```python
from build123d import *

# Parameters (mm, degrees)
F1_DEPTH = 3
F2_DEPTH = 6
F3_W     = 3
F3_H     = 2.9
F4_DEPTH = 1.5
F5_DEPTH = 3
F6_R     = 0.5


with BuildPart() as f1:
    # F0 (on Top) → F1 (new body)
    with BuildSketch(Plane.XY):
        with BuildLine():
            Line((-8.1, -17.1), (8.1, -17.1))
            ThreePointArc((8.1, -17.1), (14.463961, -14.463961), (17.1, -8.1))
            Line((17.1, -8.1), (17.1, 8.1))
            ThreePointArc((17.1, 8.1), (14.463961, 14.463961), (8.1, 17.1))
            Line((8.1, 17.1), (-8.1, 17.1))
            ThreePointArc((-8.1, 17.1), (-14.463961, 14.463961), (-17.1, 8.1))
            Line((-17.1, 8.1), (-17.1, -8.1))
            ThreePointArc((-17.1, -8.1), (-14.463961, -14.463961), (-8.1, -17.1))
        make_face()
        with BuildLine():
            ThreePointArc((14, -6.1), (12.974874, -8.574874), (10.5, -9.6))
            Line((10.5, -9.6), (-10.5, -9.6))
            ThreePointArc((-10.5, -9.6), (-12.974874, -8.574874), (-14, -6.1))
            Line((-14, -6.1), (-14, 0))
            Line((-14, 0), (-14, 8.1))
            ThreePointArc((-14, 8.1), (-12.242641, 12.342641), (-8, 14.1))
            Line((-8, 14.1), (8, 14.1))
            ThreePointArc((8, 14.1), (12.242641, 12.342641), (14, 8.1))
            Line((14, 8.1), (14, 0))
            Line((14, 0), (14, -6.1))
        make_face(mode=Mode.SUBTRACT)
    extrude(amount=F1_DEPTH)

    # F0 (on Top) → F2 (join)
    with BuildSketch(Plane.XY):
        with BuildLine():
            Line((-20, -20), (20, -20))
            Line((20, -20), (20, 9.5))
            ThreePointArc((20, 9.5), (16.924621, 16.924621), (9.5, 20))
            Line((9.5, 20), (-9.5, 20))
            ThreePointArc((-9.5, 20), (-16.924621, 16.924621), (-20, 9.5))
            Line((-20, 9.5), (-20, -20))
        make_face()
        with BuildLine():
            ThreePointArc((17.1, -8.1), (14.463961, -14.463961), (8.1, -17.1))
            Line((8.1, -17.1), (-8.1, -17.1))
            ThreePointArc((-8.1, -17.1), (-14.463961, -14.463961), (-17.1, -8.1))
            Line((-17.1, -8.1), (-17.1, 8.1))
            ThreePointArc((-17.1, 8.1), (-14.463961, 14.463961), (-8.1, 17.1))
            Line((-8.1, 17.1), (8.1, 17.1))
            ThreePointArc((8.1, 17.1), (14.463961, 14.463961), (17.1, 8.1))
            Line((17.1, 8.1), (17.1, -8.1))
        make_face(mode=Mode.SUBTRACT)
    extrude(amount=F2_DEPTH)

    # F3 (on face) → F4 (cut)
    with BuildSketch(Plane.XY.offset(3)):
        Polygon((1.5, -17.1), (4.25, -17.1), (4.25, -9.6), (-4.25, -9.6), (-4.25, -17.1), (-1.5, -17.1), align=None)
        with Locations((0, -18.55)):
            Rectangle(F3_W, F3_H)
    extrude(amount=-F4_DEPTH, mode=Mode.SUBTRACT)

    # F3 (on face) → F5 (cut, through all)
    with BuildSketch(Plane.XY.offset(3)):
        with Locations((0, -18.55)):
            Rectangle(F3_W, F3_H)
    extrude(amount=F5_DEPTH, mode=Mode.SUBTRACT)

    # F6
    f6_edges = [f1.edges().sort_by_distance(p)[0] for p in [
        (-14.463961, 14.463961, 6),
        (-1.5, -18.55, 6),
        (1.5, -18.55, 6),
        (-4.25, -13.35, 3),
        (4.25, -13.35, 3),
    ]]
    fillet(f6_edges, radius=F6_R)


solid = f1.part
```
Can you work these out from the model? Positions are in its coordinate system, mm. A direction names the side the tool comes from. Coordinates: 2 decimals unless noted, no trailing zeros. Loops run counter-clockwise (first coordinate to the right, second up) from the corner with the lowest first, then second, coordinate; pieces in that order, holes last. Notation, with made-up numbers: (-19, -10.5) -> (9, -10.5) arc R19 cw to (9, 3.5) -> close; hole circle Ø3 at (51.25, 76). An arc over 180 degrees is marked (long way). Put each result on its own line as item: value. Start each with the question number.
Q1. For faces 5 (the face through (-12.289, 12.296, 1.479)), 6 (the face through (-1.5, -19, 4)), 7 (the face through (14.394, 14.534, 4.232)), which set-ups out of +Z, -Z, +X, -X, +Y, -Y let a thin tool reach every point of the face, with its end or its side?
Q2. Thinking about a two-plate mould opening in Y: for faces 1 (the face through (0, 14.1, 1)), 2 (the face through (1.5, -19, 3)), 3 (the face through (12.196, 12.389, 1.479)), 4 (the face through (-16.84, 17.01, 2.96)), which applies, pulls with the +Y half, pulls with the -Y half, needs draft (parallel to the pull), parting line crosses it, or undercut?
Q3. I'm going to push a flat-ended pin straight in: P1, Ø6, axis at x = -4.5, y = 13, coming from the -Z side. Where does the tip first touch, or does it pass through?
Q4. I want a section at C-C (z = 5). Write out the boundary of the cut face in (x, y).
Q5. I want a section at D-D (z = 2). Write out the boundary of the cut face in (x, y), plus the area to 3 significant figures.
Q6. If I drill on line 1 (Y direction, x = 5, z = 4.25); line 2 (X direction, y = 6, z = 0.75); line 3 (Y direction, x = 5, z = 1), over which ranges is the centre line in solid material (lowest first)? Write a range as [from, to].
Q7. I want a section at A-A (x = -3). Write out the boundary of the cut face in (y, z), plus the area to 3 significant figures.
Q8. I want a section at B-B (y = -3.5). Write out the boundary of the cut face in (x, z), plus the area to 3 significant figures.
Taken from the geometry:
1. face 5: +Z, -Z
1. face 6: +Z, -Y
1. face 7: +Z
2. face 1: undercut
2. face 2: needs draft
2. face 3: undercut
2. face 4: pulls with the +Y half
3. P1: stops at z = 0
4. outline: (-20, -20) -> (-1.5, -20) -> (-1.5, -17.1) -> (-8.1, -17.1) arc R9 cw to (-17.1, -8.1) -> (-17.1, 8.1) arc R9 cw to (-8.1, 17.1) -> (8.1, 17.1) arc R9 cw to (17.1, 8.1) -> (17.1, -8.1) arc R9 cw to (8.1, -17.1) -> (1.5, -17.1) -> (1.5, -20) -> (20, -20) -> (20, 9.5) arc R10.5 ccw to (9.5, 20) -> (-9.5, 20) arc R10.5 ccw to (-20, 9.5) -> close
5. outline: (-20, -20) -> (-1.5, -20) -> (-1.5, -17.1) -> (-4.25, -17.1) -> (-4.25, -9.6) -> (-10.5, -9.6) arc R3.5 cw to (-14, -6.1) -> (-14, 8.1) arc R6 cw to (-8, 14.1) -> (8, 14.1) arc R6 cw to (14, 8.1) -> (14, -6.1) arc R3.5 cw to (10.5, -9.6) -> (4.25, -9.6) -> (4.25, -17.1) -> (1.5, -17.1) -> (1.5, -20) -> (20, -20) -> (20, 9.5) arc R10.5 ccw to (9.5, 20) -> (-9.5, 20) arc R10.5 ccw to (-20, 9.5) -> close
5. area: 837 mm2
6. line 1: y = [-20, -17.1], [17.1, 20]
6. line 2: x = [-20, -14], [14, 20]
6. line 3: y = [-20, -9.6], [14.1, 20]
7. outline: (-20, 0) -> (-9.6, 0) -> (-9.6, 1.5) -> (-17.1, 1.5) -> (-17.1, 5.5) arc R0.5 ccw to (-17.6, 6) -> (-20, 6) -> close; (14.1, 0) -> (20, 0) -> (20, 6) -> (17.6, 6) arc R0.5 ccw to (17.1, 5.5) -> (17.1, 3) -> (14.1, 3) -> close
7. area: 54.9 mm2
8. outline: (-20, 0) -> (-14, 0) -> (-14, 3) -> (-17.1, 3) -> (-17.1, 5.5) arc R0.5 ccw to (-17.6, 6) -> (-20, 6) -> close; (14, 0) -> (20, 0) -> (20, 6) -> (17.6, 6) arc R0.5 ccw to (17.1, 5.5) -> (17.1, 3) -> (14, 3) -> close
8. area: 53.3 mm2
